```python
from build123d import *

# Parameters (mm, degrees)
F0_W      = 108.4
F0_H      = 24.4
F0_R      = 1
F0_R_2    = 4.1
F1_DEPTH  = 1.5
F2_W      = 108.4
F2_H      = 1.5
F3_DEPTH  = 15
F4_W      = 22.2
F4_H      = 15
F5_DEPTH  = 1.5
F7_R      = 2
F8_R      = 5
F9_W      = 32
F9_H      = 1.5
F10_DEPTH = 13
F6_R      = 1
F11_DEPTH = 1.5
F12_R     = 1
F13_DEPTH = 1.5
F14_R     = 2


with BuildPart() as f1:
    # F0 (on Top) → F1 (new body)
    with BuildSketch(Plane.XY):
        Rectangle(F0_W, F0_H)
        with Locations((-51.2, -7.2)):
            Circle(F0_R, mode=Mode.SUBTRACT)
        with Locations((-19.6, -7.2)):
            Circle(F0_R, mode=Mode.SUBTRACT)
        with Locations((19.6, -7.2)):
            Circle(F0_R, mode=Mode.SUBTRACT)
        with Locations((51.2, -7.2)):
            Circle(F0_R, mode=Mode.SUBTRACT)
        with Locations((-45, 0)):
            Circle(F0_R_2, mode=Mode.SUBTRACT)
        with BuildLine():
            ThreePointArc((-37.5, 4.8), (-36.0355339059, 8.3355339059), (-32.5, 9.8))
            Line((-32.5, 9.8), (-22.8, 9.8))
            ThreePointArc((-22.8, 9.8), (-22.0928932188, 9.5071067812), (-21.8, 8.8))
            Line((-21.8, 8.8), (-21.8, 5.5901699437))
            ThreePointArc((-21.8, 5.5901699437), (-21.7128709292, 5.1819216533), (-21.4666666667, 4.8448139512))
            ThreePointArc((-21.4666666667, 4.8448139512), (-19.3, 0), (-21.4666666667, -4.8448139512))
            ThreePointArc((-21.4666666667, -4.8448139512), (-21.7128709292, -5.1819216533), (-21.8, -5.5901699437))
            Line((-21.8, -5.5901699437), (-21.8, -8.8))
            ThreePointArc((-21.8, -8.8), (-22.0928932188, -9.5071067812), (-22.8, -9.8))
            Line((-22.8, -9.8), (-32.5, -9.8))
            ThreePointArc((-32.5, -9.8), (-36.0355339059, -8.3355339059), (-37.5, -4.8))
            Line((-37.5, -4.8), (-37.5, 4.8))
        make_face(mode=Mode.SUBTRACT)
        with Locations((-51.2, 7.2)):
            Circle(F0_R, mode=Mode.SUBTRACT)
        with Locations((-19.6, 7.2)):
            Circle(F0_R, mode=Mode.SUBTRACT)
        with BuildLine():
            Line((21.8, 5.5901699437), (21.8, 8.8))
            ThreePointArc((21.8, 8.8), (22.0928932188, 9.5071067812), (22.8, 9.8))
            Line((22.8, 9.8), (32.5, 9.8))
            ThreePointArc((32.5, 9.8), (36.0355339059, 8.3355339059), (37.5, 4.8))
            Line((37.5, 4.8), (37.5, -4.8))
            ThreePointArc((37.5, -4.8), (36.0355339059, -8.3355339059), (32.5, -9.8))
            Line((32.5, -9.8), (22.8, -9.8))
            ThreePointArc((22.8, -9.8), (22.0928932188, -9.5071067812), (21.8, -8.8))
            Line((21.8, -8.8), (21.8, -5.5901699437))
            ThreePointArc((21.8, -5.5901699437), (21.7128709292, -5.1819216533), (21.4666666667, -4.8448139512))
            ThreePointArc((21.4666666667, -4.8448139512), (19.3, 0), (21.4666666667, 4.8448139512))
            ThreePointArc((21.4666666667, 4.8448139512), (21.7128709292, 5.1819216533), (21.8, 5.5901699437))
        make_face(mode=Mode.SUBTRACT)
        with Locations((45, 0)):
            Circle(F0_R_2, mode=Mode.SUBTRACT)
        with Locations((19.6, 7.2)):
            Circle(F0_R, mode=Mode.SUBTRACT)
        with Locations((51.2, 7.2)):
            Circle(F0_R, mode=Mode.SUBTRACT)
    extrude(amount=F1_DEPTH)

    # F2 (on face) → F3 (join)
    with BuildSketch(Plane.XZ.offset(12.2)):
        with Locations((0, 0.75)):
            Rectangle(F2_W, F2_H)
    extrude(amount=F3_DEPTH)

    # F4 (on face) → F5 (cut, through all)
    with BuildSketch(Plane.XY.offset(1.5)):
        with Locations((-43.1, -19.7)):
            Rectangle(F4_W, F4_H)
        with Locations((43.1, -19.7)):
            Rectangle(F4_W, F4_H)
    extrude(amount=-F5_DEPTH, mode=Mode.SUBTRACT)

    # F7
    f7_edges = [f1.edges().sort_by_distance(p)[0] for p in [
        (-32, -12.2, 0.75),
        (32, -12.2, 0.75),
    ]]
    fillet(f7_edges, radius=F7_R)

    # F8
    f8_edges = [f1.edges().sort_by_distance(p)[0] for p in [
        (-54.2, 12.2, 0.75),
        (-54.2, -12.2, 0.75),
        (54.2, 12.2, 0.75),
        (54.2, -12.2, 0.75),
    ]]
    fillet(f8_edges, radius=F8_R)

    # F9 (on face) → F10 (join)
    with BuildSketch(Plane(origin=(0, 12.2, 0), x_dir=(-1, 0, 0), z_dir=(0, 1, 0))):
        with Locations((-16, 0.75)):
            Rectangle(F9_W, F9_H)
        with Locations((16, 0.75)):
            Rectangle(F9_W, F9_H)
    extrude(amount=F10_DEPTH)

    # F6 (on face) → F11 (cut, through all)
    with BuildSketch(Plane.XY.offset(1.5)):
        with Locations((-10, -24.2)):
            Circle(F6_R)
        with Locations((10, -24.2)):
            Circle(F6_R)
    extrude(amount=-F11_DEPTH, mode=Mode.SUBTRACT)

    # F12 (on face) → F13 (cut, through all)
    with BuildSketch(Plane.XY.offset(1.5)):
        with Locations((-23.5, 20.5)):
            Circle(F12_R)
        with Locations((23.5, 20.5)):
            Circle(F12_R)
        with Locations((-23.5, -22.5)):
            Circle(F12_R)
        with Locations((23.5, -22.5)):
            Circle(F12_R)
        with Locations((-29.5, 15)):
            Circle(F12_R)
        with Locations((-29.5, -17)):
            Circle(F12_R)
        with Locations((29.5, 15)):
            Circle(F12_R)
        with Locations((29.5, -17)):
            Circle(F12_R)
    extrude(amount=-F13_DEPTH, mode=Mode.SUBTRACT)

    # F14
    f14_edges = [f1.edges().sort_by_distance(p)[0] for p in [
        (-32, -27.2, 0.75),
        (32, -27.2, 0.75),
        (32, 25.2, 0.75),
        (32, 12.2, 0.75),
        (-32, 12.2, 0.75),
        (-32, 25.2, 0.75),
    ]]
    fillet(f14_edges, radius=F14_R)


solid = f1.part
```
Could you check a few things on this model? Use its own coordinates, in mm. A direction names the side the tool comes from. Give positions to 0.01 mm unless a question says otherwise; leave off trailing zeros. Write each loop counter-clockwise with the first axis right and the second up, starting at its lowest first coordinate (ties: lowest second). Pieces come first, ordered by that corner, then holes. Notation, with made-up numbers: (36.25, 10.5) -> (67.25, 10.5) arc R24 cw to (67.25, 41.5) -> close; hole circle Ø10 at (-0.5, 7.25). An arc over 180 degrees is marked (long way). Write each question's results on one line, items separated by ' | '.
1. I want a section at A-A, the plane y = 20.5. Write out the boundary of the cut face in (x, z), then the cut area to 3 significant figures.
Check sheet entries:
outline: (-32, 0) -> (-24.5, 0) -> (-24.5, 1.5) -> (-32, 1.5) -> close; (-22.5, 0) -> (22.5, 0) -> (22.5, 1.5) -> (-22.5, 1.5) -> close; (24.5, 0) -> (32, 0) -> (32, 1.5) -> (24.5, 1.5) -> close | area: 90.0 mm²
2. I want a section at D-D, the plane z = 0.6. Count the separate pieces of the cut face and the enclosed holes in it, then the cut area to 3 significant figures.
Check sheet entries:
separate pieces: 1 | enclosed holes: 22 | area: 3,620 mm²
3. If we mould it in two halves opening along X, with no side actions, what happens to faces 3 (the flat face through (-1, -1, 0)), 4 (the cylindrical face through (32.57, 12.8, 0.76)), 5 (the cylindrical face through (-49.096, 0.18, 0.74))? For each: released by +X, released by -X, zero draft, split by the parting line, or undercut.
Check sheet entries:
face 3: zero draft | face 4: released by +X | face 5: undercut
4. I need wall thicknesses on L1, parallel to Y at x = 29.5, z = 1.1; L2, parallel to Y at x = -45, z = 0.3; L3, parallel to Y at x = -51.2, z = 0.6. Which ranges of each line are inside material? Lowest first, please.
Check sheet entries:
L1: y = -27.2 to -18, -16 to -9.8, 9.8 to 14, 16 to 25.2 | L2: y = -12.2 to -4.1, 4.1 to 12.2 | L3: y = -11.78 to -8.2, -6.2 to 6.2, 8.2 to 11.78
5. I want a section at C-C, the plane x = 51.2. Write out the boundary of the cut face in (y, z), then the cut area to 3 significant figures.
Check sheet entries:
outline: (-11.78, 0) -> (-8.2, 0) -> (-8.2, 1.5) -> (-11.78, 1.5) -> close; (-6.2, 0) -> (6.2, 0) -> (6.2, 1.5) -> (-6.2, 1.5) -> close; (8.2, 0) -> (11.78, 0) -> (11.78, 1.5) -> (8.2, 1.5) -> close | area: 29.3 mm²
6. On a 3-axis mill with a long thin cutter (end or side, diameter ignored), from which of +Z, -Z, +X, -X, +Y, -Y can I reach the whole of each face in a straight line? I mean faces 1 (the cylindrical face through (-52.77, 10.7, 0.76)), 2 (the cylindrical face through (-36.07, 8.3, 0.74)). Say none if no direction works.
Check sheet entries:
face 1: +Z, -Z, -X, +Y | face 2: +Z, -Z
7. Will this pin go through, and if not, where does the flat tip stop? pin 1 Ø1.2 at (x, y) = (-51.2, 7.2) entering from +Z.
Check sheet entries:
pin 1: passes through
8. I want a section at B-B, the plane y = 0. Write out the boundary of the cut face in (x, z), then the cut area to 3 significant figures.
Check sheet entries:
outline: (-54.2, 0) -> (-49.1, 0) -> (-49.1, 1.5) -> (-54.2, 1.5) -> close; (-40.9, 0) -> (-37.5, 0) -> (-37.5, 1.5) -> (-40.9, 1.5) -> close; (-19.3, 0) -> (19.3, 0) -> (19.3, 1.5) -> (-19.3, 1.5) -> close; (37.5, 0) -> (40.9, 0) -> (40.9, 1.5) -> (37.5, 1.5) -> close; (49.1, 0) -> (54.2, 0) -> (54.2, 1.5) -> (49.1, 1.5) -> close | area: 83.4 mm²
